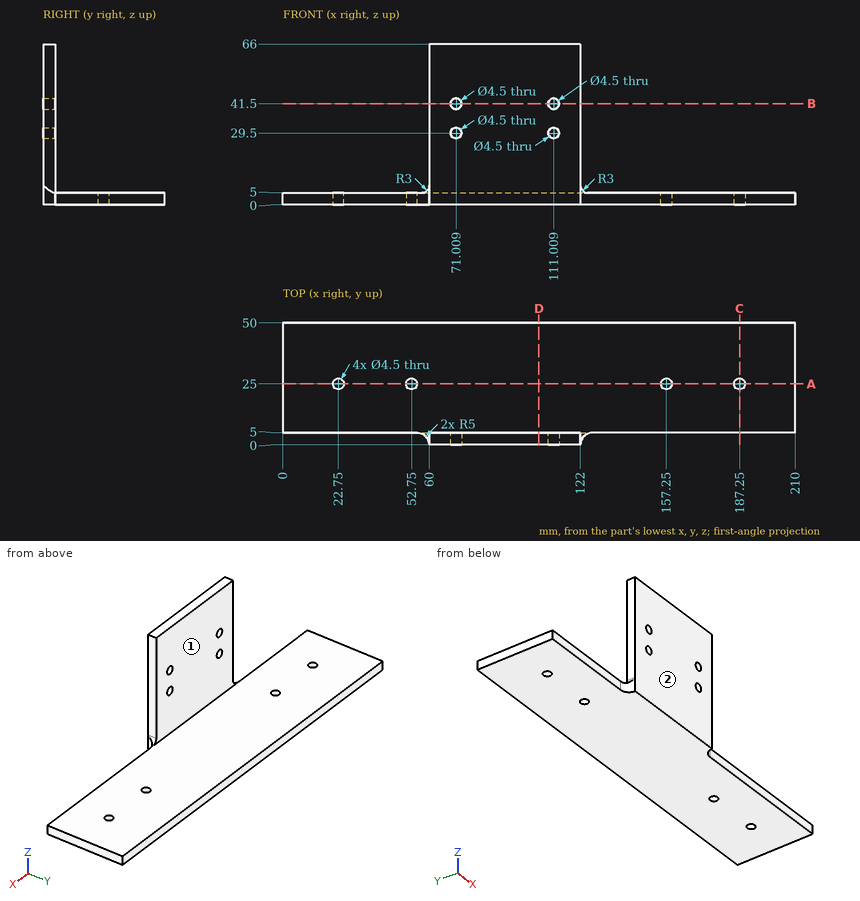
Source: three-view drawing plus pictorial views. Frame: mm from the lowest corner of the part. A direction names the side the tool comes from. Give positions to 0.01 mm unless a question says otherwise; leave off trailing zeros. Order: outer loops, then holes, each group sorted by start corner. A loop starts at its lowest first (then second) coordinate and runs counter-clockwise, first axis right, second up. Notation, with made-up numbers: (65.25, 68.25) -> (104.25, 68.25) arc R26 cw to (104.25, 98.25) -> close; hole circle Ø9 at (29, 9.25). An arc over 180 degrees is marked (long way). Put each result on its own line as item: value.
Q1. Pin query (flat end, axial travel): pin 1 (22.5 mm diameter, centred on x = 97.5, y = 28.5, fed in from +Z); pin 2 (18.5 mm diameter, centred on x = 76.5, z = 34.5, fed in from +Y); pin 3 (2.5 mm diameter, centred on x = 183, z = 2, fed in from -Y). Return the tip coordinate at first contact, or that it passes through.
Here are the results:
pin 1: stops at z = 5
pin 2: stops at y = 5
pin 3: stops at y = 5
Q2. Section C-C, the plane x = 187.25. Return loops of the section in (y, z).
Here are the results:
outline: (5, 0) -> (22.75, 0) -> (22.75, 5) -> (5, 5) -> close; (27.25, 0) -> (50, 0) -> (50, 5) -> (27.25, 5) -> close
Q3. Material intervals for L1, parallel to Y at x = 157.25, z = 3.3; L2, parallel to Z at x = 87.5, y = 12, sorted ascending.
Here are the results:
L1: y = 5 to 22.75, 27.25 to 50
L2: z = 0 to 5
Q4. Reachability of the marked faces 1 and 2 from +Z, -Z, +X, -X, +Y, -Y: full face, straight path, thin tool, end or side. Return the list, or none.
Here are the results:
face 1: +Z, +X, -X, +Y
face 2: +Z, -Z, +X, -X, -Y
Q5. Section D-D, the plane x = 105. Return loops of the section in (y, z).
Here are the results:
outline: (0, 0) -> (50, 0) -> (50, 5) -> (5, 5) -> (5, 66) -> (0, 66) -> close
Q6. Section B-B, the plane z = 41.5. Return loops of the section in (x, y).
Here are the results:
outline: (60, 0) -> (68.76, 0) -> (68.76, 5) -> (60, 5) -> close; (73.26, 0) -> (108.76, 0) -> (108.76, 5) -> (73.26, 5) -> close; (113.26, 0) -> (122, 0) -> (122, 5) -> (113.26, 5) -> close
Q7. Section A-A, the plane y = 25. Return loops of the section in (x, z).
Here are the results:
outline: (0, 0) -> (20.5, 0) -> (20.5, 5) -> (0, 5) -> close; (25, 0) -> (50.5, 0) -> (50.5, 5) -> (25, 5) -> close; (55, 0) -> (155, 0) -> (155, 5) -> (55, 5) -> close; (159.5, 0) -> (185, 0) -> (185, 5) -> (159.5, 5) -> close; (189.5, 0) -> (210, 0) -> (210, 5) -> (189.5, 5) -> close
